The listing builds one solid part. Answer for the finished solid, in the listing's coordinates (mm). A direction names the side the tool comes from. Coordinates: 2 decimals unless noted, no trailing zeros. Order: outer loops, then holes, each group sorted by start corner. A loop starts at its lowest first (then second) coordinate and runs counter-clockwise, first axis right, second up. Notation, with made-up numbers: (60.25, 43.25) -> (79.25, 43.25) arc R33 ccw to (79.25, 82.25) -> close; hole circle Ø7 at (13, 54). An arc over 180 degrees is marked (long way). Return JSON: item names as keys, results as strings.
```python
from build123d import *

# Parameters (mm, degrees)
BOSS_EXTRUDE1_DEPTH = 10


with BuildPart() as part:
    # Sketch1 → Boss-Extrude1 (new body)
    with BuildSketch(Plane(origin=(0, 0, 0), x_dir=(1, 0, 0), z_dir=(0, 1, 0))):
        with BuildLine():
            Line((0, -116.07), (56.57, -116.07))
            ThreePointArc((56.57, -116.07), (98.642853481, -98.642853481), (116.07, -56.57))
            Line((116.07, -56.57), (116.07, 0))
            Line((116.07, 0), (103.07, 0))
            Line((103.07, 0), (103.07, -3))
            Line((103.07, -3), (110.57, -3))
            Line((110.57, -3), (110.57, -56.57))
            ThreePointArc((110.57, -56.57), (94.753766184, -94.753766184), (56.57, -110.57))
            Line((56.57, -110.57), (3, -110.57))
            Line((3, -110.57), (3, -103.07))
            Line((3, -103.07), (0, -103.07))
            Line((0, -103.07), (0, -116.07))
        make_face()
    extrude(amount=BOSS_EXTRUDE1_DEPTH)


solid = part.part
```
Item 1: The part is cut by section D-D on z = 9. Determine the outline of the cut face in (x, y).
Answer list:
{"outline": "(110.57, 0) -> (116.07, 0) -> (116.07, 10) -> (110.57, 10) -> close"}
Item 2: Determine the mould class of faces 5 (the flat face through (107, 5, 3)), 6 (the flat face through (116.07, 5, 29)), 7 (the cylindrical face through (98.18, 4.93, 99.1)) for opening direction Z: pulls with the +Z half, pulls with the -Z half, needs draft (parallel to the pull), parting line crosses it, or undercut.
Answer list:
{"face 5": "undercut", "face 6": "needs draft", "face 7": "pulls with the +Z half"}
Item 3: Which of the six approach directions +Z, -Z, +X, -X, +Y, -Y give full straight-line access (tool end or side, diameter ignored) to faces 1 (the flat face through (110.57, 5, 29)), 2 (the cylindrical face through (95.2, 4.9, 94.3)), 3 (the flat face through (2, 5, 103.07)), 4 (the flat face through (3, 5, 107))?
Answer list:
{"face 1": "-X, +Y, -Y", "face 2": "+Y, -Y", "face 3": "-Z, -X, +Y, -Y", "face 4": "-Z, +Y, -Y"}
Item 4: Find the intervals of material crossed by probe 1 along X at (y, z) = (1.5, 49.5); probe 2 along X at (y, z) = (3, 66.5), in increasing order.
Answer list:
{"probe 1": "110.57 to 116.07", "probe 2": "109.65 to 115.24"}
Item 5: The part is cut by section B-B on y = 7.75. Determine the outline of the cut face in (x, z), plus the area to 3 significant figures.
Answer list:
{"outline": "(0, 103.07) -> (3, 103.07) -> (3, 110.57) -> (56.57, 110.57) arc R54 cw to (110.57, 56.57) -> (110.57, 3) -> (103.07, 3) -> (103.07, 0) -> (116.07, 0) -> (116.07, 56.57) arc R59.5 ccw to (56.57, 116.07) -> (0, 116.07) -> close", "area": "1,160 mm2"}
Item 6: Flat-ended cylindrical pins translate along their axes: pin 1 (2 mm diameter, centred on y = 3, z = 106, fed in from +X); pin 2 (3 mm diameter, centred on x = 27.5, y = 3.5, fed in from -Z); pin 3 (0.9 mm diameter, centred on x = 1, y = 5, fed in from -Z). Find the tip coordinate at first contact, or state that the pin passes through.
Answer list:
{"pin 1": "x = 91.14", "pin 2": "z = 110.57", "pin 3": "z = 103.07"}
Item 7: The part is cut by section C-C on x = 41. Determine the outline of the cut face in (y, z), plus the area to 3 significant figures.
Answer list:
{"outline": "(0, 110.57) -> (10, 110.57) -> (10, 116.07) -> (0, 116.07) -> close", "area": "55.0 mm2"}
Item 8: The part is cut by section A-A on z = 106. Determine the outline of the cut face in (x, y), plus the area to 3 significant figures.
Answer list:
{"outline": "(0, 0) -> (3, 0) -> (3, 10) -> (0, 10) -> close; (78.31, 0) -> (89.69, 0) -> (89.69, 10) -> (78.31, 10) -> close", "area": "144 mm2"}
